Can you work these out from the model? Positions are in its coordinate system, mm. Face numbers are marked on the shaded views. A direction names the side the tool comes from. Give positions to 0.01 mm unless a question says otherwise; leave off trailing zeros. Loops run counter-clockwise (first coordinate to the right, second up) from the corner with the lowest first, then second, coordinate; pieces in that order, holes last. Notation, with made-up numbers: (7.5, 49.5) - (16.5, 49.5) arc R26 ccw to (16.5, 79.5) - close; hole circle Ø7 at (20, 31.5). An arc over 180 degrees is marked (long way). Answer as a JSON object with one key per item and string values.
Autodesk Inventor part; units mm, degrees
ref_plane "YZ Plane" through (0, 0, 0) normal (1, 0, 0) x (0, 1, 0)
ref_plane "XZ Plane" through (0, 0, 0) normal (0, 1, 0) x (-1, 0, 0)
ref_plane "XY Plane" through (0, 0, 0) normal (0, 0, 1) x (1, 0, 0)
sketch "Sketch1" plane through (0, 0, 0) normal (1, 0, 0) x (0, 1, 0)
  line L0 (0, 0) -> (25.4, 0)
  line L1 (25.4, 0) -> (28.575, 0)
  line L2 (28.575, 0) -> (28.575, -12.7)
  line L3 (28.575, -12.7) -> (25.4, -12.7)
  line L4 (25.4, -12.7) -> (25.4, 0)
  line L5 (28.575, 0) -> (28.575, 12.7)
  line L6 (28.575, 12.7) -> (0, 0)
  dimension "d0" = 25.4
  dimension "d1" = 3.175
  dimension "d2" = 12.7
  dimension "d3" = 12.7
extrude "Extrusion1" add sketch "Sketch1" along normal blind 53.34
sketch "Sketch2" plane through (0, 28.575, 12.7) normal (0, 1, 0) x (1, 0, 0)
  line L0 (53.34, 25.4) -> (53.34, 19.05)
  line L1 (53.34, 25.4) -> (53.34, 0)
  line L2 (53.34, 19.05) -> (26.67, 19.05)
  circle A0 centre (26.67, 19.05) radius 2.1082
  point P0 (0, 12.7)
  dimension "d6" = 6.35
  dimension "d7" = 26.67
  dimension "d8" = 4.2164
extrude "Extrusion2" cut sketch "Sketch2" against normal blind 43.815
sketch "Sketch3" plane through (53.34, 0, 0) normal (1, 0, 0) x (0, 0, -1)
  line L0 (12.7, 25.4) -> (12.7, 28.575)
  line L1 (12.7, 28.575) -> (-16.4619, 28.575)
  line L2 (-16.4619, 28.575) -> (-16.4619, 0)
  line L3 (-16.4619, 0) -> (12.7, 0)
  line L4 (12.7, 0) -> (12.7, 28.575)
  point P0 (0, 0)
extrude "Extrusion3" cut sketch "Sketch3" against normal blind 20.32
sketch "Sketch4" plane through (0, 28.575, 12.7) normal (0, 1, 0) x (1, 0, 0)
  circle A0 centre (26.67, 19.05) radius 2.1082
  line L0 (26.67, 19.05) -> (13.97, 19.05)
  circle A1 centre (13.97, 19.05) radius 2.1082
  point P0 (0, 12.7)
  dimension "d13" = 12.7
extrude "Extrusion4" cut sketch "Sketch4" against normal blind 20.32 contours A1
properties part number "sleds v2"
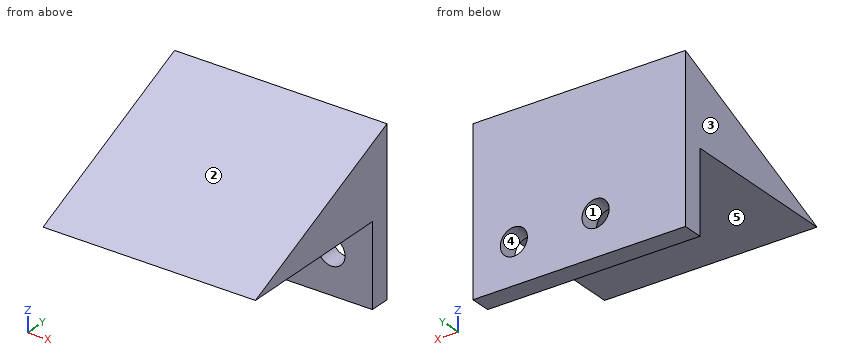
1) I'm going to push flat-ended pins straight in: P1, Ø7.5, axis at x = 11, y = 18.5, coming from the -Z side; P2, Ø3, axis at x = 20, y = 3.5, coming from the +Z side; P3, Ø5, axis at x = 11.5, y = 24.5, coming from the +Z side; P4, Ø4, axis at x = 13.97, z = -6.35, coming from the -Y side. Where does each tip first touch, or does it pass through?
Check sheet entries:
{"P1": "z = 0", "P2": "z = 2.22", "P3": "z = 12", "P4": "through"}
2) Imagine slicing it at D-D on y = 22.5. Write out the boundary of the cut face in (x, z).
Check sheet entries:
{"outline": "(0, 0) - (33.02, 0) - (33.02, 10) - (0, 10) - close"}
3) Imagine slicing it at B-B on z = -6.35. Write out the boundary of the cut face in (x, y) (3 decimals).
Check sheet entries:
{"outline": "(0, 25.4) - (11.862, 25.4) - (11.862, 28.575) - (0, 28.575) - close; (16.078, 25.4) - (24.562, 25.4) - (24.562, 28.575) - (16.078, 28.575) - close; (28.778, 25.4) - (33.02, 25.4) - (33.02, 28.575) - (28.778, 28.575) - close"}
4) Imagine slicing it at A-A on x = 13.97. Write out the boundary of the cut face in (y, z) (3 decimals).
Check sheet entries:
{"outline": "(0, 0) - (25.4, 0) - (25.4, -4.242) - (28.575, -4.242) - (28.575, 12.7) - close; (25.4, -12.7) - (28.575, -12.7) - (28.575, -8.458) - (25.4, -8.458) - close"}
5) Which directions (+Z, -Z, +X, -X, +Y, -Y) give clear straight access to the entire face, cutting with the end or side of a thin tool? Please do the marked faces 4 and 5.
Check sheet entries:
{"face 4": "+Y, -Y", "face 5": "-Z, +X, -X, -Y"}
6) Imagine slicing it at C-C on x = 6. Write out the boundary of the cut face in (y, z) (3 decimals), and give its area (3 significant figures).
Check sheet entries:
{"outline": "(0, 0) - (25.4, 0) - (25.4, -12.7) - (28.575, -12.7) - (28.575, 12.7) - close", "area": "222 mm2"}
7) If we mould it in two halves opening along X, with no side actions, what happens to the marked faces 1, 2 and 3? For each: released by +X, released by -X, zero draft, split by the parting line, or undercut.
Check sheet entries:
{"face 1": "undercut", "face 2": "zero draft", "face 3": "released by -X"}
8) I need wall thicknesses on L1, parallel to X at y = 26.2, z = -6.35; L2, parallel to Y at x = 17.5, z = -9.75 (3 decimals); L3, parallel to Z at x = 13.97, y = 26.7. Which ranges of each line are inside material? Lowest first, please.
Check sheet entries:
{"L1": "0 to 11.86, 16.08 to 24.56, 28.78 to 33.02", "L2": "25.4 to 28.575", "L3": "-12.7 to -8.46, -4.24 to 11.87"}
